Build history of the part. All positions in model axes, mm. A direction names the side the tool comes from. Coordinates: 2 decimals unless noted, no trailing zeros. Write each loop counter-clockwise with the first axis right and the second up, starting at its lowest first coordinate (ties: lowest second). Pieces come first, ordered by that corner, then holes.
from build123d import *
from build123d.topology import SkipClean

# Parameters (mm, degrees)
SKETCH1_R           = 14.5415
BOSS_EXTRUDE2_DEPTH = 2.54
BOSS_EXTRUDE4_START = 2.54
SKETCH1_8_W         = 3.81
SKETCH1_8_H         = 3.81
BOSS_EXTRUDE4_DEPTH = 1
BOSS_EXTRUDE3_START = 2.54
SKETCH1_6_R         = 14.5415
BOSS_EXTRUDE3_DEPTH = 1.9
SKETCH1_9_R         = 1.5875
CUT_EXTRUDE2_DEPTH  = 3.175
SKETCH2_R           = 14.5415
SKETCH2_R_2         = 12.954
BOSS_EXTRUDE5_DEPTH = 1.5
BOSS_EXTRUDE6_DEPTH = 3.4
FILLET1_R           = 1
CHAMFER1_SIZE       = 0.635
CUT_EXTRUDE3_DEPTH  = 22.405467631
CIRPATTERN1_COUNT   = 4


with BuildPart() as part:
    # Sketch1 → Boss-Extrude2 (new body)
    with BuildSketch(Plane(origin=(0, 0, 0), x_dir=(1, 0, 0), z_dir=(0, 1, 0))):
        with Locations(Location((0, 0, 0), (0, 0, 270))):
            Circle(SKETCH1_R)
    extrude(amount=BOSS_EXTRUDE2_DEPTH)

    # Sketch1<8> → Boss-Extrude4 (add)
    with BuildSketch(Plane(origin=(0, 0, 0), x_dir=(1, 0, 0), z_dir=(0, 1, 0)).offset(BOSS_EXTRUDE4_START)):
        Rectangle(SKETCH1_8_W, SKETCH1_8_H)
    extrude(amount=BOSS_EXTRUDE4_DEPTH)

    # Sketch1<6> → Boss-Extrude3 (add)
    with BuildSketch(Plane(origin=(0, 0, 0), x_dir=(1, 0, 0), z_dir=(0, 1, 0)).offset(BOSS_EXTRUDE3_START)):
        with Locations(Location((0, 0, 0), (0, 0, 90))):
            Circle(SKETCH1_6_R)
        with BuildLine():
            ThreePointArc((6.096, -11.43), (8.929053506, -9.384994379), (11.1125, -6.657211109))
            Line((11.1125, -6.657211109), (11.1125, 6.657211109))
            ThreePointArc((11.1125, 6.657211109), (8.363458286, 9.8923547), (4.716130935, 12.065))
            Line((4.716130935, 12.065), (-4.716130935, 12.065))
            ThreePointArc((-4.716130935, 12.065), (-8.363458286, 9.8923547), (-11.1125, 6.657211109))
            Line((-11.1125, 6.657211109), (-11.1125, -6.657211109))
            ThreePointArc((-11.1125, -6.657211109), (-8.929053506, -9.384994379), (-6.096, -11.43))
            Line((-6.096, -11.43), (6.096, -11.43))
        make_face(mode=Mode.SUBTRACT)
    extrude(amount=BOSS_EXTRUDE3_DEPTH)

    # Sketch1<9> → Cut-Extrude2 (cut)
    with BuildSketch(Plane(origin=(0, 0, 0), x_dir=(1, 0, 0), z_dir=(0, 1, 0))):
        with Locations(Location((0, 0, 0), (0, 0, 270))):
            Circle(SKETCH1_9_R)
        with Locations(Location((-5.461, 3.81, 0), (0, 0, 270))):
            Circle(SKETCH1_9_R)
        with Locations(Location((5.461, 3.81, 0), (0, 0, 270))):
            Circle(SKETCH1_9_R)
        with Locations(Location((5.461, -3.81, 0), (0, 0, 270))):
            Circle(SKETCH1_9_R)
        with Locations(Location((-5.461, -3.81, 0), (0, 0, 270))):
            Circle(SKETCH1_9_R)
    extrude(amount=CUT_EXTRUDE2_DEPTH, mode=Mode.SUBTRACT)

    # Sketch2 → Boss-Extrude5 (add)
    with BuildSketch(Plane(origin=(0, 4.44, 0), x_dir=(1, 0, 0), z_dir=(0, 1, 0))):
        with Locations(Location((0, 0, 0), (0, 0, 270))):
            Circle(SKETCH2_R)
        with Locations(Location((0, 0, 0), (0, 0, 68.649791106))):
            Circle(SKETCH2_R_2, mode=Mode.SUBTRACT)
    extrude(amount=BOSS_EXTRUDE5_DEPTH)

    # Sketch3 → Boss-Extrude6 (add)
    with BuildSketch(Plane(origin=(0, 2.54, 0), x_dir=(1, 0, 0), z_dir=(0, 1, 0))):
        with BuildLine():
            Line((-10.657411412, 7.363810019), (-7.363810019, 7.363810019))
            Line((-7.363810019, 7.363810019), (-7.363810019, 10.657411412))
            ThreePointArc((-7.363810019, 10.657411412), (-9.159861243, 9.159861243), (-10.657411412, 7.363810019))
        make_face()
        with BuildLine():
            Line((-10.657411412, -7.363810019), (-7.363810019, -7.363810019))
            Line((-7.363810019, -7.363810019), (-7.363810019, -10.657411412))
            ThreePointArc((-7.363810019, -10.657411412), (-9.159861243, -9.159861243), (-10.657411412, -7.363810019))
        make_face()
    extrude(amount=BOSS_EXTRUDE6_DEPTH)

    # Fillet1
    fillet1_edges = [part.edges().sort_by_distance(p)[0] for p in [
        (1.905, 3.04, -1.905),
        (-1.905, 3.04, -1.905),
        (-1.905, 3.04, 1.905),
        (1.905, 3.04, 1.905),
    ]]
    fillet(fillet1_edges, radius=FILLET1_R)

    # Chamfer1
    chamfer1_edges = [part.edges().sort_by_distance(p)[0] for p in [
        (-7.363810019, 4.24, 7.363810019),
        (-7.363810019, 4.24, -7.363810019),
    ]]
    chamfer(chamfer1_edges, length=CHAMFER1_SIZE)

    # Sketch4 → Cut-Extrude3 (cut, symmetric)
    with SkipClean():  # the faces are left unmerged after this step: merging them gives an invalid solid
        with BuildSketch(Plane.XY):
            Polygon((-14.5415, 2.765), (-13.74775, 2.765), (-13.74775, 1.635771776), (-14.5415, 1.1775), align=None)
        cut_extrude3 = extrude(amount=CUT_EXTRUDE3_DEPTH, both=True, mode=Mode.SUBTRACT)

    # CirPattern1: Cut-Extrude3 ×4 about axis
    with SkipClean():  # the faces are left unmerged after this step: merging them gives an invalid solid
        cirpattern1_axis = Axis((0, 0, 0), (0, 1, 0))
        for i in range(1, CIRPATTERN1_COUNT):
            add(cut_extrude3.rotate(cirpattern1_axis, i * 360 / CIRPATTERN1_COUNT), mode=Mode.SUBTRACT)


solid = part.part
(1) 3-axis set-ups, long thin cutter, end or side, ignore diameter. For faces 1 (the cylindrical face through (-0.966, 1.565, -1.26)), 2 (the cylindrical face through (4.495, 1.252, -5.07)), 3 (the flat face through (0, 3, -12.065)): which of +Z, -Z, +X, -X, +Y, -Y reach the whole face in a straight line?
(2) Slice it at C-C, the plane x = 0. List the corners of the cut face in (y, z) (1 decimal), and give its area (3 significant figures).
(3) Slice it at A-A, the plane y = 4.8. List the corners of the cut face in (x, z), and give its area (3 significant figures).
(4) Two-plate mould, pull along X, no slides. Class faces 4 (the cylindrical face through (4.05, 1.25, 4.54)), 5 (the flat face through (-1.905, 3, 0)), 6 (the flat face through (0, 2, -13.748)): pulls with the +X half, pulls with the -X half, needs draft (parallel to the pull), parting line crosses it, or undercut.
(5) Flat gauge pins, fed straight in: P1, Ø0.6, axis at x = -2, y = 2, coming from the -Z side; P2, Ø1.3, axis at y = 3.5, z = -9.5, coming from the +X side; P3, Ø2, axis at x = -11, z = 3, coming from the +Y side. Where does each tip first touch, or does it go through?
(6) Slice it at B-B, the plane z = -3.81. Give the number of separate pieces and of enclosed holes in the cut face, and give its area (3 significant figures).
(7) Probe L1, parallel to Z at x = 0.25, y = 4.5; L2, parallel to X at y = 1, z = 3.81; L3, parallel to Z at x = 6.75, y = 1.45. List the from-to ranges inside material, lowest first.
(8) Slice it at D-D, the plane y = 2. List the corners of the cut face in (x, z) (1 decimal).
Results:
1. face 1: -Y
1. face 2: +Y, -Y
1. face 3: +Y
2. outline: (0, -14.5) - (1.2, -14.5) - (1.6, -13.7) - (2.8, -13.7) - (2.8, -14.5) - (5.9, -14.5) - (5.9, -13) - (4.4, -13) - (4.4, -12.1) - (2.5, -12.1) - (2.5, -1.9) - (3.5, -1.9) - (3.5, 1.9) - (2.5, 1.9) - (2.5, 11.4) - (4.4, 11.4) - (4.4, 13) - (5.9, 13) - (5.9, 14.5) - (2.8, 14.5) - (2.8, 13.7) - (1.6, 13.7) - (1.2, 14.5) - (0, 14.5) - (0, 1.6) - (3.2, 1.6) - (3.2, -1.6) - (0, -1.6) - close
2. area: 80.8 mm2
3. outline: circle Ø29.08 at (0, 0); hole (-10.66, -7.36) - (-8, -7.36) - (-7.36, -8) - (-7.36, -10.66) arc R12.95 ccw (long way) to (-7.36, 10.66) - (-7.36, 8) - (-8, 7.36) - (-10.66, 7.36) arc R12.95 ccw to start
3. area: 149 mm2
4. face 4: undercut
4. face 5: undercut
4. face 6: needs draft
5. P1: stops at z = -13.75
5. P2: stops at x = 11.54
5. P3: stops at y = 4.44
6. separate pieces: 3
6. enclosed holes: 0
6. area: 70.5 mm2
7. L1: z = -14.54 to -12.95, 12.95 to 14.54
7. L2: x = -14.03 to -7.05, -3.87 to 3.87, 7.05 to 14.03
7. L3: z = -12.88 to -4.74, -2.88 to 2.88, 4.74 to 12.88
8. outline: (-13.7, -4.7) arc R14.5 ccw to (-4.7, -13.7) - (4.7, -13.7) arc R14.5 ccw to (13.7, -4.7) - (13.7, 4.7) arc R14.5 ccw to (4.7, 13.7) - (-4.7, 13.7) arc R14.5 ccw to (-13.7, 4.7) - close; hole circle Ø3.2 at (-5.5, -3.8); hole circle Ø3.2 at (-5.5, 3.8); hole circle Ø3.2 at (0, 0); hole circle Ø3.2 at (5.5, -3.8); hole circle Ø3.2 at (5.5, 3.8)
